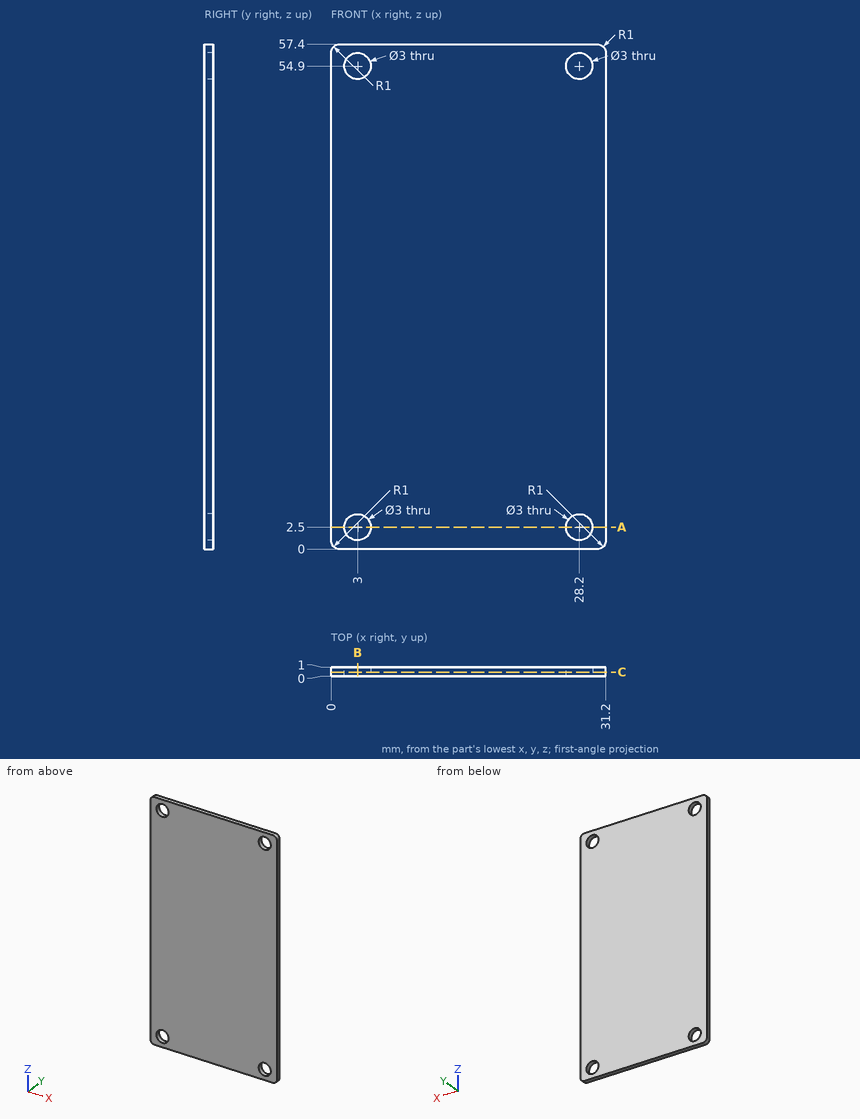
Answer from the drawing. Dimensions are ordinates in mm from the lowest x, y and z of the part. Coordinates: 2 decimals unless noted, no trailing zeros. Order: outer loops, then holes, each group sorted by start corner. A loop starts at its lowest first (then second) coordinate and runs counter-clockwise, first axis right, second up. Notation, with made-up numbers: (-28, 79.5) - (1, 79.5) arc R25 ccw to (1, 115.5) - close; hole circle Ø4 at (6, 45.25). An arc over 180 degrees is marked (long way). Put each result on its own line as item: value. Start each with the question number.
1) Find the intervals of material crossed by line 1 (Z direction, x = 3, y = 0.35); line 2 (Z direction, x = 27.5, y = 0.85), in increasing order. Write a range as from..to.
2) Find section C-C (y = 0.45). Give the vertices of the cut face in (x, z).
3) Find section A-A (z = 2.5). Give the vertices of the cut face in (x, y), plus the area to 3 significant figures.
4) Find section B-B (x = 3). Give the vertices of the cut face in (y, z), plus the area to 3 significant figures.
Results list:
1. line 1: z = 0..1, 4..53.4, 56.4..57.4
1. line 2: z = 0..1.17, 3.83..53.57, 56.23..57.4
2. outline: (0, 1) arc R1 ccw to (1, 0) - (30.2, 0) arc R1 ccw to (31.2, 1) - (31.2, 56.4) arc R1 ccw to (30.2, 57.4) - (1, 57.4) arc R1 ccw to (0, 56.4) - close; hole circle Ø3 at (3, 2.5); hole circle Ø3 at (3, 54.9); hole circle Ø3 at (28.2, 2.5); hole circle Ø3 at (28.2, 54.9)
3. outline: (0, 0) - (1.5, 0) - (1.5, 1) - (0, 1) - close; (4.5, 0) - (26.7, 0) - (26.7, 1) - (4.5, 1) - close; (29.7, 0) - (31.2, 0) - (31.2, 1) - (29.7, 1) - close
3. area: 25.2 mm^2
4. outline: (0, 0) - (1, 0) - (1, 1) - (0, 1) - close; (0, 4) - (1, 4) - (1, 53.4) - (0, 53.4) - close; (0, 56.4) - (1, 56.4) - (1, 57.4) - (0, 57.4) - close
4. area: 51.4 mm^2
